```python
from build123d import *

# Parameters (mm, degrees)
PAD_DEPTH     = 2
SKETCH003_W   = 6.666667
SKETCH003_H   = 3
SKETCH003_W_2 = 6.666666
SKETCH003_W_3 = 3
SKETCH003_H_2 = 10
PAD001_DEPTH  = 12


with BuildPart() as part:
    # AdditivePipe: sweep along a path in Sketch
    with BuildLine(Plane.XY) as additivepipe_path:
        Line((-40, 15), (-40, -15))
        ThreePointArc((-40, -15), (-37.071068, -22.071068), (-30, -25))
        Line((-30, -25), (30, -25))
        ThreePointArc((30, -25), (37.071068, -22.071068), (40, -15))
        Line((40, -15), (40, 15))
        ThreePointArc((40, 15), (37.071068, 22.071068), (30, 25))
        Line((30, 25), (-30, 25))
        ThreePointArc((-30, 25), (-37.071068, 22.071068), (-40, 15))
    # Sketch002 → AdditivePipe (sweep)
    with BuildSketch(Plane.YZ):
        Polygon((-25, 0), (-28, 0), (-25, 2), align=None)
    sweep(path=additivepipe_path.line)

    # Sketch001 → Pad (new body)
    with BuildSketch(Plane.XY):
        with BuildLine():
            Line((-40, 15), (-40, -15))
            ThreePointArc((-40, -15), (-37.071068, -22.071068), (-30, -25))
            Line((-30, -25), (30, -25))
            ThreePointArc((30, -25), (37.071068, -22.071068), (40, -15))
            Line((40, -15), (40, 15))
            ThreePointArc((40, 15), (37.071068, 22.071068), (30, 25))
            Line((30, 25), (-30, 25))
            ThreePointArc((-30, 25), (-37.071068, 22.071068), (-40, 15))
        make_face()
    extrude(amount=PAD_DEPTH)

    # Sketch003 → Pad001 (join)
    with BuildSketch(Plane.XY):
        with BuildLine():
            ThreePointArc((-30, 28), (-39.192388, 24.192388), (-43, 15))
            Line((-43, 15), (-40, 15))
            ThreePointArc((-30, 25), (-37.071068, 22.071068), (-40, 15))
            Line((-30, 25), (-30, 28))
        make_face()
        with BuildLine():
            ThreePointArc((-43, -15), (-39.192388, -24.192388), (-30, -28))
            Line((-30, -28), (-30, -25))
            ThreePointArc((-40, -15), (-37.071068, -22.071068), (-30, -25))
            Line((-43, -15), (-40, -15))
        make_face()
        with BuildLine():
            ThreePointArc((30, -28), (39.192388, -24.192388), (43, -15))
            Line((40, -15), (43, -15))
            ThreePointArc((30, -25), (37.071068, -22.071068), (40, -15))
            Line((30, -28), (30, -25))
        make_face()
        with BuildLine():
            ThreePointArc((43, 15), (39.192388, 24.192388), (30, 28))
            Line((30, 25), (30, 28))
            ThreePointArc((40, 15), (37.071068, 22.071068), (30, 25))
            Line((40, 15), (43, 15))
        make_face()
        with Locations((16.666666, 26.5)):
            Rectangle(SKETCH003_W, SKETCH003_H)
        with Locations((0, 26.5)):
            Rectangle(SKETCH003_W_2, SKETCH003_H)
        with Locations((-16.666666, 26.5)):
            Rectangle(SKETCH003_W, SKETCH003_H)
        with Locations((-16.666666, -26.5)):
            Rectangle(SKETCH003_W, SKETCH003_H)
        with Locations((0, -26.5)):
            Rectangle(SKETCH003_W_2, SKETCH003_H)
        with Locations((16.666666, -26.5)):
            Rectangle(SKETCH003_W, SKETCH003_H)
        with Locations((-41.5, 0)):
            Rectangle(SKETCH003_W_3, SKETCH003_H_2)
        with Locations((41.5, 0)):
            Rectangle(SKETCH003_W_3, SKETCH003_H_2)
    extrude(amount=PAD001_DEPTH)


solid = part.part
```
The model under review builds one solid part; all positions refer to its coordinate system, in mm. A direction names the side the tool comes from. Coordinates: 2 decimals unless noted, no trailing zeros. Write each loop counter-clockwise with the first axis right and the second up, starting at its lowest first coordinate (ties: lowest second). Pieces come first, ordered by that corner, then holes. Notation, with made-up numbers: (85, 38.5) - (94, 38.5) arc R27 ccw to (94, 66.5) - close; hole circle Ø1 at (32, -1.5). An arc over 180 degrees is marked (long way). Write item = value, one per line.
(1) Consider section A-A, the plane y = 20. Give the boundary of the cut face in (x, z).
Result sheet:
outline = (-42, 0) - (42, 0) - (42, 12) - (38.66, 12) - (38.66, 2) - (-38.66, 2) - (-38.66, 12) - (-42, 12) - close
(2) Consider section C-C, the plane z = 4.25. State how many separate pieces and enclosed holes the cut face has, then the cut area to 3 significant figures.
Result sheet:
separate_pieces = 12
enclosed_holes = 0
area = 397 mm^2
(3) Mouldability with a two-part tool opening along Y and no side actions: class faces 1 (the face through (17, 25, 7)), 2 (the face through (-40, 0, 7)), 3 (the face through (0, -26, 12)), 4 (the face through (0, 28, 6)) as pulls with the +Y half, pulls with the -Y half, needs draft (parallel to the pull), parting line crosses it, or undercut.
Result sheet:
face_1 = undercut
face_2 = undercut
face_3 = needs draft
face_4 = pulls with the +Y half
(4) Machinability: for faces 5 (the face through (-41.5, -10.1, 1)), 6 (the face through (41, 15, 6)), 7 (the face through (0, 25, 7)), 8 (the face through (-3.333, 26, 6)), which of the approach directions +Z, -Z, +X, -X, +Y, -Y give a long, thin tool a straight path to every point of the face, cutting with its end or side? Answer none if there is none.
Result sheet:
face_5 = +Z, -X
face_6 = +Z, +X
face_7 = +Z
face_8 = +Z, +Y
(5) Consider section D-D, the plane x = -25. Give the boundary of the cut face in (y, z).
Result sheet:
outline = (-28, 0) - (28, 0) - (25, 2) - (-25, 2) - close
(6) For line 1 (Y direction, x = 16, z = 6.5); line 2 (X direction, y = -4.5, z = 4.5); line 3 (Z direction, x = -31, y = -2.5), list the stretches that pass through material, from the lowest coordinate up. Write a range as [from, to].
Result sheet:
line_1 = [-28, -25], [25, 28]
line_2 = [-43, -40], [40, 43]
line_3 = [0, 2]
(7) Consider section B-B, the plane x = -34.5. Give the boundary of the cut face in (y, z), then the cut area to 3 significant figures.
Result sheet:
outline = (-27.2, 0) - (27.2, 0) - (27.2, 12) - (23.93, 12) - (23.93, 2) - (-23.93, 2) - (-23.93, 12) - (-27.2, 12) - close
area = 174 mm^2
(8) For P1, Ø6, axis at x = 27.5, y = -13.5, coming from the +Z side; P2, Ø3.5, axis at y = 27, z = 5.5, coming from the -X side; P3, Ø0.9, axis at y = -26, z = 4, coming from the -X side, all flat-tipped, find the tip position at first contact; note any pin that passes through.
Result sheet:
P1 = 2
P2 = -38
P3 = -37.6
